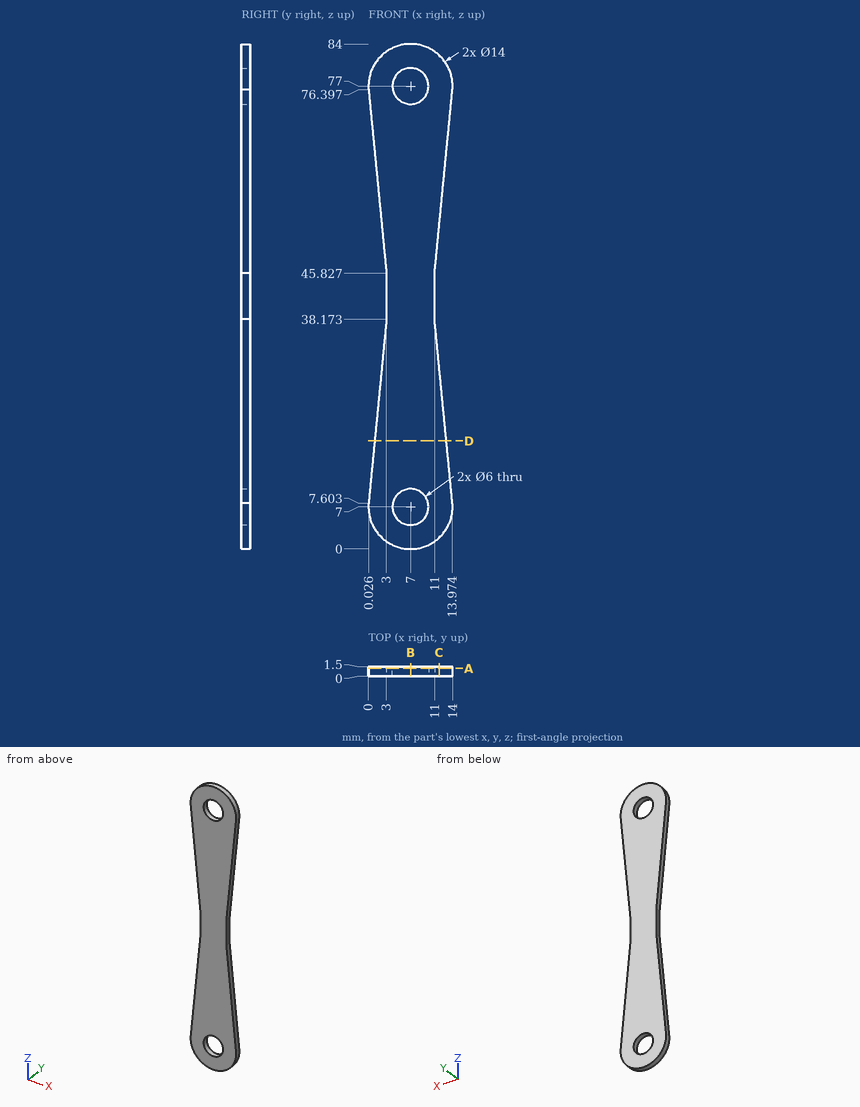
Can you work these out from the drawing? Everything is in mm from the part's minimum corner. Round coordinates to 2 decimals unless told otherwise and drop trailing zeros. Loops run counter-clockwise (first coordinate to the right, second up) from the corner with the lowest first, then second, coordinate; pieces in that order, holes last. Notation, with made-up numbers: M 56,-36.75 L 106,-36.75 A16 cw 106,-20.75 Z; hole C 33.5,49 d1. An arc over 180 degrees is marked long. Answer in a Markdown table with one row per item.
1. Please list where these lines run through material, in increasing order: line 1 (Z direction, x = 7, y = 0.8); line 2 (Z direction, x = 4.25, y = 0.75) (1 decimal); line 3 (X direction, y = 1.15, z = 5.5). Write a range as from..to.
Established:
| item | result |
|---|---|
| line 1 | 0..4, 10..74, 80..84 |
| line 2 | 0.6..5.8, 8.2..75.8, 78.2..83.4 |
| line 3 | 0.16..4.4, 9.6..13.84 |
2. If we section it at A-A, the plane y = 1.25: Please give me the cut outline in (x, z).
Established:
| item | result |
|---|---|
| outline | M 0.03,7.6 A7 ccw long 13.97,7.6 L 11,38.17 L 11,45.83 L 13.97,76.4 A7 ccw long 0.03,76.4 L 3,45.83 L 3,38.17 Z; hole C 7,7 d6; hole C 7,77 d6 |
3. If we section it at C-C, the plane x = 11.75: Please give me the cut outline in (y, z).
Established:
| item | result |
|---|---|
| outline | M 0,1.86 L 1.5,1.86 L 1.5,30.46 L 0,30.46 Z; M 0,53.54 L 1.5,53.54 L 1.5,82.14 L 0,82.14 Z |
4. I'm going to push flat-ended pins straight in: pin 1 Ø5.5 at (x, z) = (7, 7) entering from +Y; pin 2 Ø0.8 at (y, z) = (0.5, 43.5) entering from -X; pin 3 Ø8 at (x, z) = (7, 77) entering from -Y; pin 4 Ø0.8 at (y, z) = (0.5, 41.5) entering from +X. Where does each tip first touch, or does it pass through?
Established:
| item | result |
|---|---|
| pin 1 | through |
| pin 2 | x = 3 |
| pin 3 | y = 0 |
| pin 4 | x = 11 |
5. If we section it at B-B, the plane x = 7: Please give me the cut outline in (y, z), plus the area to 3 significant figures.
Established:
| item | result |
|---|---|
| outline | M 0,0 L 1.5,0 L 1.5,4 L 0,4 Z; M 0,10 L 1.5,10 L 1.5,74 L 0,74 Z; M 0,80 L 1.5,80 L 1.5,84 L 0,84 Z |
| area | 108 mm² |
6. If we section it at D-D, the plane z = 18: Please give me the cut outline in (x, y).
Established:
| item | result |
|---|---|
| outline | M 1.04,0 L 12.96,0 L 12.96,1.5 L 1.04,1.5 Z |
